```python
from build123d import *

# Parameters (mm, degrees)
F1_DEPTH = 17.5
F2_R     = 4
F3_DEPTH = 25
F4_R     = 4.4
F5_DEPTH = 25
F6_R     = 2


# Not quite as in the source:
# - a feature names something its author has since deleted; it is built from what else it names


with BuildPart() as f1:
    # F0 (on Front) → F1 (new body, symmetric)
    with BuildSketch(Plane.XZ):
        Polygon((95, -38), (95, 15), (-95, 15), (-95, -38), (-115, -38), (-115, -40), (-93, -40), (-93, 13), (93, 13), (93, -40), (115, -40), (115, -38), align=None)
    extrude(amount=F1_DEPTH, both=True)

    # F2 (on face) → F3 (cut)
    with BuildSketch(Plane.XY.offset(-38)):
        with Locations((-105, 0)):
            Circle(F2_R)
        with Locations((105, 0)):
            Circle(F2_R)
    extrude(amount=-F3_DEPTH, mode=Mode.SUBTRACT)

    # F4 (on face) → F5 (cut)
    with BuildSketch(Plane.XY.offset(15)):
        with Locations((-32.5, 0)):
            Circle(F4_R)
        with Locations((32.5, 0)):
            Circle(F4_R)
    extrude(amount=-F5_DEPTH, mode=Mode.SUBTRACT)

    # F6
    f6_edges = [f1.edges().sort_by_distance(p)[0] for p in [
        (95, 0, 15),
        (-95, 0, 15),
        (-93, 0, -40),
        (93, 0, -40),
    ]]
    fillet(f6_edges, radius=F6_R)


solid = f1.part
```
Part model, mm, in its own coordinate system. A direction names the side the tool comes from. Round coordinates to 2 decimals unless told otherwise and drop trailing zeros. Order: outer loops, then holes, each group sorted by start corner. A loop starts at its lowest first (then second) coordinate and runs counter-clockwise, first axis right, second up. Notation, with made-up numbers: M 21,15 L 39,15 A34 cw 39,46 Z; hole C 64.5,-26.75 d4. An arc over 180 degrees is marked long. Put each result on its own line as item: value. Start each with the question number.
1. Slice it at A-A on x = 32.5. List the corners of the cut face in (y, z).
2. Two-plate mould, pull along Y, no slides. Class faces 1 (the face through (-109, 0, -39)), 2 (the face through (107, -4, -40)), 3 (the face through (-1, 17.5, 14)): +Y half, -Y half, draft (parallel to the pull), parting line (faces both ways), or undercut.
3. Slice it at D-D on y = 14. List the corners of the cut face in (x, z), then the cut area to 3 significant figures.
4. Tool access for faces 4 (the face through (-93, 0, -13)), 5 (the face through (-95, 0, -12)), 6 (the face through (95, 0, -13)), 7 (the face through (36.564, -1.685, 14.014)): list every direction of +Z, -Z, +X, -X, +Y, -Y with a clear straight run to the whole face (end or side of a thin tool).
5. Slice it at B-B on y = 0. State how many separate pieces and enclosed holes the cut face has, then the cut area to 3 significant figures.
6. Drill centre lines: probe 1 along X at (y, z) = (1.5, 12.5); probe 2 along Y at (x, z) = (32, 14); probe 3 along Y at (x, z) = (105, -38.85). Where is each one in solid material? Low to high. Write a range as [from, to].
7. Slice it at C-C on z = -34. List the corners of the cut face in (x, y), then the cut area to 3 significant figures.
8. Drop flat-ended pins along their axis: pin 1 (11.5 mm diameter, centred on x = 32.5, y = 0, fed in from +Z); pin 2 (4 mm diameter, centred on x = 6.5, y = 3.5, fed in from -Z); pin 3 (5 mm diameter, centred on x = -105, y = 0, fed in from +Z); pin 4 (3 mm diameter, centred on y = -8, z = -23.5, fed in from +X). Give the stop position or say it passes through.
Findings:
1. outline: M -17.5,13 L -4.4,13 L -4.4,15 L -17.5,15 Z; M 4.4,13 L 17.5,13 L 17.5,15 L 4.4,15 Z
2. face 1: undercut
2. face 2: draft
2. face 3: +Y half
3. outline: M -115,-40 L -95,-40 A2 ccw -93,-38 L -93,13 L 93,13 L 93,-38 A2 ccw 95,-40 L 115,-40 L 115,-38 L 95,-38 L 95,13 A2 ccw 93,15 L -93,15 A2 ccw -95,13 L -95,-38 L -115,-38 Z
3. area: 669 mm2
4. face 4: -Z, +Y, -Y
4. face 5: +Z, -X, +Y, -Y
4. face 6: +Z, +X, +Y, -Y
4. face 7: +Z, -Z
5. separate pieces: 5
5. enclosed holes: 0
5. area: 601 mm2
6. probe 1: [-95, -93], [93, 95]
6. probe 2: [-17.5, -4.37], [4.37, 17.5]
6. probe 3: [-17.5, -4], [4, 17.5]
7. outline: M -95,-17.5 L -93,-17.5 L -93,17.5 L -95,17.5 Z; M 93,-17.5 L 95,-17.5 L 95,17.5 L 93,17.5 Z
7. area: 140 mm2
8. pin 1: z = 15
8. pin 2: z = 13
8. pin 3: through
8. pin 4: x = 95
